Answer from the drawing. Dimensions are ordinates in mm from the lowest x, y and z of the part. Give positions to 0.01 mm unless a question says otherwise; leave off trailing zeros. Loops run counter-clockwise (first coordinate to the right, second up) from the corner with the lowest first, then second, coordinate; pieces in that order, holes last. Notation, with made-up numbers: M 81,-13.75 L 87,-13.75 A19 cw 87,4.25 Z; hole C 52.5,64.5 d8. An arc over 180 degrees is marked long. Use a Markdown table: item, result.
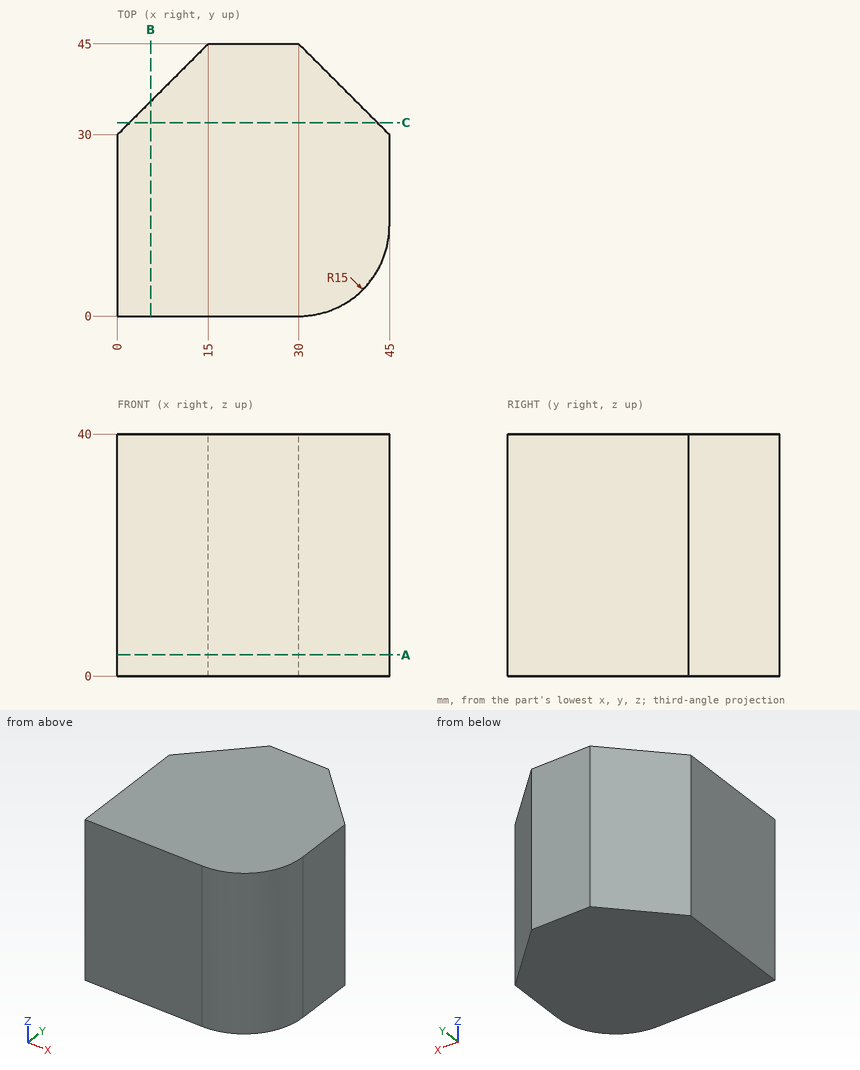
(1) A cutting plane is placed at A-A (z = 3.5). Write down the section's boundary in (x, y).
Entries:
| item | result |
|---|---|
| outline | M 0,0 L 30,0 A15 ccw 45,15 L 45,30 L 30,45 L 15,45 L 0,30 Z |
(2) A cutting plane is placed at B-B (x = 5.5). Write down the section's boundary in (y, z).
Entries:
| item | result |
|---|---|
| outline | M 0,0 L 35.5,0 L 35.5,40 L 0,40 Z |
(3) Given P1, Ø12, axis at x = 10.5, z = 13, coming from the +Y side; P2, Ø8, axis at x = 40, z = 17, coming from the +Y side; P3, Ø6, axis at y = 36.5, z = 29, coming from the -X side; P4, Ø1, axis at x = 33.5, z = 21.5, coming from the +Y side, each flat-ended and moving along its own axis, determine where each tip first touches the part or whether it passes through.
Entries:
| item | result |
|---|---|
| P1 | stops at y = 45 |
| P2 | stops at y = 39 |
| P3 | stops at x = 3.5 |
| P4 | stops at y = 42 |
(4) A cutting plane is placed at C-C (y = 32). Write down the section's boundary in (x, z).
Entries:
| item | result |
|---|---|
| outline | M 2,0 L 43,0 L 43,40 L 2,40 Z |
(5) Consider probe 1 along X at (y, z) = (34, 37); probe 2 along Y at (x, z) = (14.5, 31); probe 3 along X at (y, z) = (9, 22). Determine where each line is inside the solid, lowest interval first. Write a range as [from, to].
Entries:
| item | result |
|---|---|
| probe 1 | x = [4, 41] |
| probe 2 | y = [0, 44.5] |
| probe 3 | x = [0, 43.75] |
